Could you check a few things on this drawing? It's one solid part, dimensions in mm from its lowest x, y, z. Give positions to 0.01 mm unless a question says otherwise; leave off trailing zeros. Order: outer loops, then holes, each group sorted by start corner. A loop starts at its lowest first (then second) coordinate and runs counter-clockwise, first axis right, second up.
Item 1: I want a section at B-B, the plane y = 18.5. Write out the boundary of the cut face in (x, z) (1 decimal).
Item 2: I want a section at A-A, the plane z = 10.16. Write out the boundary of the cut face in (x, y).
Item 3: I'm going to push flat-ended pins straight in: pin 1 Ø3 at (x, y) = (10.5, 6) entering from -Z; pin 2 Ø3 at (x, z) = (9.5, 6.5) entering from +Y; pin 3 Ø1.5 at (x, y) = (2.5, 14) entering from +Z. Where does each tip first touch, or does it pass through?
Item 4: If I drill on line 1 along Y through (x, z) = (6.75, 10.16); line 2 along Z through (x, y) = (8, 3.25) (1 decimal); line 3 along Z through (x, y) = (4.5, 8.5) (1 decimal), over which ranges is the centre line in solid material (lowest first)?
Item 5: If we mould it in two halves opening along Y, with no side actions, what happens to the marked faces 1 and 2? For each: +Y half, -Y half, draft (parallel to the pull), parting line (faces both ways), or undercut.
Item 6: I want a section at C-C, the plane z = 14.5. Write out the boundary of the cut face in (x, y) (1 decimal).
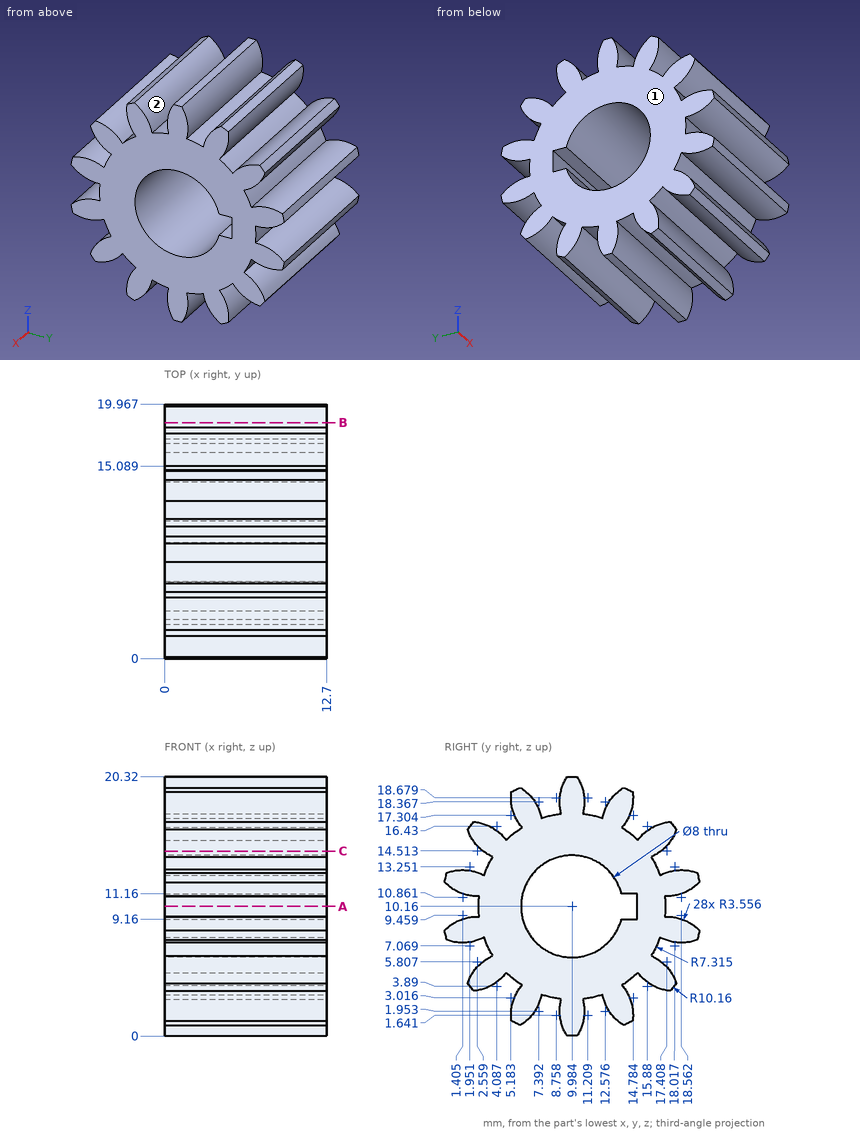
Results list:
1. outline: (0, 7.3) - (12.7, 7.3) - (12.7, 9.2) - (0, 9.2) - close; (0, 11.1) - (12.7, 11.1) - (12.7, 13) - (0, 13) - close
2. outline: (0, 2.67) - (12.7, 2.67) - (12.7, 5.98) - (0, 5.98) - close; (0, 15.09) - (12.7, 15.09) - (12.7, 17.3) - (0, 17.3) - close
3. pin 1: stops at z = 0.85
3. pin 2: stops at y = 19.91
3. pin 3: stops at z = 19.47
4. line 1: y = 2.67 to 5.98, 15.09 to 17.3
4. line 2: z = 3.8 to 6, 7.3 to 13, 14.3 to 16.6
4. line 3: z = 3 to 6.4, 13.9 to 17.3
5. face 1: draft
5. face 2: undercut
6. outline: (0, 3) - (12.7, 3) - (12.7, 17) - (0, 17) - close
